```python
from build123d import *

# Parameters (mm, degrees)
BOSS_EXTRUDE1_DEPTH = 5.842
SKETCH2_W           = 12.7
SKETCH2_H           = 3.175
CUT_EXTRUDE1_DEPTH  = 41.686011454
FILLET1_START       = -1
FILLET1_DEPTH       = 8
FILLET1_2_DEPTH     = 5.842


with BuildPart() as part:
    # Sketch1 → Boss-Extrude1 (new body)
    with BuildSketch(Plane.XY):
        Polygon((0, 0), (-25.4, 0), (-25.4, 6.35), (-31.242, 6.35), (-31.242, 19.05), (-25.4, 19.05), (-25.4, 25.4), (0, 25.4), (0, 19.05), (5.842, 19.05), (5.842, 6.35), (0, 6.35), align=None)
    extrude(amount=BOSS_EXTRUDE1_DEPTH)

    # Sketch2 → Cut-Extrude1 (cut, through all)
    with BuildSketch(Plane.XY.offset(5.842)):
        with Locations((-12.7, 23.8125)):
            Rectangle(SKETCH2_W, SKETCH2_H)
        with Locations((-12.7, 1.5875)):
            Rectangle(SKETCH2_W, SKETCH2_H)
    extrude(amount=-CUT_EXTRUDE1_DEPTH, mode=Mode.SUBTRACT)

    # Fillet1: read off the stored shape, not the designer's step
    # Fillet1 outline → Fillet1 (cut)
    with BuildSketch(Plane.XY.offset(FILLET1_START)):
        with BuildLine():
            ThreePointArc((-20.6375, 25.4), (-19.514967985, 24.935032015), (-19.05, 23.8125))
            Line((-19.05, 23.8125), (-19.05, 25.4))
            Line((-19.05, 25.4), (-20.6375, 25.4))
        make_face()
        with BuildLine():
            Line((-6.35, 25.4), (-6.35, 23.8125))
            ThreePointArc((-6.35, 23.8125), (-5.885032015, 24.935032015), (-4.7625, 25.4))
            Line((-4.7625, 25.4), (-6.35, 25.4))
        make_face()
        with BuildLine():
            ThreePointArc((-4.7625, 0), (-5.885032015, 0.464967985), (-6.35, 1.5875))
            Line((-6.35, 1.5875), (-6.35, 0))
            Line((-6.35, 0), (-4.7625, 0))
        make_face()
        with BuildLine():
            Line((-19.05, 0), (-19.05, 1.5875))
            ThreePointArc((-19.05, 1.5875), (-19.514967985, 0.464967985), (-20.6375, 0))
            Line((-20.6375, 0), (-19.05, 0))
        make_face()
    extrude(amount=FILLET1_DEPTH, mode=Mode.SUBTRACT)

    # Fillet1 2 outline → Fillet1 2 (add)
    with BuildSketch(Plane.XY):
        with BuildLine():
            Line((-19.05, 22.225), (-17.4625, 22.225))
            ThreePointArc((-17.4625, 22.225), (-18.585032015, 22.689967985), (-19.05, 23.8125))
            Line((-19.05, 23.8125), (-19.05, 22.225))
        make_face()
        with BuildLine():
            ThreePointArc((-6.35, 23.8125), (-6.814967985, 22.689967985), (-7.9375, 22.225))
            Line((-7.9375, 22.225), (-6.35, 22.225))
            Line((-6.35, 22.225), (-6.35, 23.8125))
        make_face()
        with BuildLine():
            Line((-6.35, 3.175), (-7.9375, 3.175))
            ThreePointArc((-7.9375, 3.175), (-6.814967985, 2.710032015), (-6.35, 1.5875))
            Line((-6.35, 1.5875), (-6.35, 3.175))
        make_face()
        with BuildLine():
            ThreePointArc((-19.05, 1.5875), (-18.585032015, 2.710032015), (-17.4625, 3.175))
            Line((-17.4625, 3.175), (-19.05, 3.175))
            Line((-19.05, 3.175), (-19.05, 1.5875))
        make_face()
    extrude(amount=FILLET1_2_DEPTH)


solid = part.part
```
Check sheet for the modelled part. Datum: model origin and axes. Units: mm. A direction names the side the tool comes from. Coordinates: 2 decimals unless noted, no trailing zeros. Loops run counter-clockwise (first coordinate to the right, second up) from the corner with the lowest first, then second, coordinate; pieces in that order, holes last.
1) Sectioned sample at C-C (y = 5.75). Record the boundary of the cut face in (x, z), and give its area (3 significant figures).
2) Access from +Z, -Z, +X, -X, +Y, -Y to the whole of each face (thin tool, end or side, straight path). Record for faces 1 (the face through (-25.4, 3, 3)), 2 (the face through (3, 6.35, 3)), 3 (the face through (-25.4, 22, 3)), 4 (the face through (0, 22, 3)).
3) Release check for a two-part mould opening along X. For faces 5 (the face through (-13, 22.225, 3)), 6 (the face through (-13, 3.175, 3)), 7 (the face through (-28, 19.05, 3)), 8 (the face through (0, 3, 3)) record: released by +X, released by -X, zero draft, split by the parting line, or undercut.
4) Material ranges on probe 1 along X at (y, z) = (1.75, 3.35); probe 2 along X at (y, z) = (3, 0.7); probe 3 along X at (y, z) = (3.75, 3.2), recorded low to high.
5) Sectioned sample at B-B (x = -10). Record the boundary of the cut face in (y, z) (3 decimals).
6) Gauge pin test, flat ends, axial feed: pin 1 (3 mm diameter, centred on y = 21.5, z = 2.5, fed in from +X); pin 2 (1.8 mm diameter, centred on y = 21, z = 1.5, fed in from -X); pin 3 (3 mm diameter, centred on x = -15, z = 1.5, fed in from +Y) (3 decimals). Record the tip position at first contact, or that the pin passes through.
Check sheet entries:
1. outline: (-25.4, 0) - (0, 0) - (0, 5.84) - (-25.4, 5.84) - close
1. area: 148 mm2
2. face 1: +Z, -Z, -X, -Y
2. face 2: +Z, -Z, +X, -Y
2. face 3: +Z, -Z, -X, +Y
2. face 4: +Z, -Z, +X, +Y
3. face 5: undercut
3. face 6: undercut
3. face 7: zero draft
3. face 8: released by +X
4. probe 1: x = -25.4 to -19.04, -6.36 to 0
4. probe 2: x = -25.4 to -18.19, -7.21 to 0
4. probe 3: x = -25.4 to 0
5. outline: (3.175, 0) - (22.225, 0) - (22.225, 5.842) - (3.175, 5.842) - close
6. pin 1: stops at x = 0
6. pin 2: stops at x = -25.4
6. pin 3: stops at y = 22.225
